```python
from build123d import *

# Parameters (mm, degrees)
SKETCH1_R           = 20
BOSS_EXTRUDE1_DEPTH = 35
CUT_EXTRUDE1_DEPTH  = 15
SKETCH3_R           = 4.1
CUT_EXTRUDE2_DEPTH  = 21
SKETCH4_R           = 2
CUT_EXTRUDE3_DEPTH  = 36
SKETCH5_R           = 17
CUT_EXTRUDE4_DEPTH  = 5
CUT_EXTRUDE5_DEPTH  = 2


with BuildPart() as part:
    # Sketch1 → Boss-Extrude1 (new body)
    with BuildSketch(Plane(origin=(0, 0, 0), x_dir=(1, 0, 0), z_dir=(0, 1, 0))):
        Circle(SKETCH1_R)
    extrude(amount=BOSS_EXTRUDE1_DEPTH)

    # Sketch2 → Cut-Extrude1 (cut)
    with BuildSketch(Plane(origin=(0, 35, 0), x_dir=(1, 0, 0), z_dir=(0, 1, 0))):
        Polygon((-8, 7.5), (-14.495190528, 3.75), (-14.495190528, -3.75), (-8, -7.5), (-1.504809472, -3.75), (-1.504809472, 3.75), align=None)
        Polygon((8, 7.5), (1.504809472, 3.75), (1.504809472, -3.75), (8, -7.5), (14.495190528, -3.75), (14.495190528, 3.75), align=None)
    extrude(amount=-CUT_EXTRUDE1_DEPTH, mode=Mode.SUBTRACT)

    # Sketch3 → Cut-Extrude2 (cut, through all)
    with BuildSketch(Plane(origin=(0, 20, 0), x_dir=(1, 0, 0), z_dir=(0, 1, 0))):
        with Locations((-8, 0)):
            Circle(SKETCH3_R)
        with Locations((8, 0)):
            Circle(SKETCH3_R)
    extrude(amount=-CUT_EXTRUDE2_DEPTH, mode=Mode.SUBTRACT)

    # Sketch4 → Cut-Extrude3 (cut, through all)
    with BuildSketch(Plane(origin=(0, 35, 0), x_dir=(1, 0, 0), z_dir=(0, 1, 0))):
        with Locations((-10.5, 10.5)):
            Circle(SKETCH4_R)
        with Locations((10.5, 10.5)):
            Circle(SKETCH4_R)
        with Locations((10.5, -10.5)):
            Circle(SKETCH4_R)
        with Locations((-10.5, -10.5)):
            Circle(SKETCH4_R)
    extrude(amount=-CUT_EXTRUDE3_DEPTH, mode=Mode.SUBTRACT)

    # Sketch5 → Cut-Extrude4 (cut)
    with BuildSketch(Plane(origin=(0, 35, 0), x_dir=(1, 0, 0), z_dir=(0, 1, 0))):
        Circle(SKETCH5_R)
    extrude(amount=-CUT_EXTRUDE4_DEPTH, mode=Mode.SUBTRACT)

    # Sketch6 → Cut-Extrude5 (cut)
    with BuildSketch(Plane.XZ):
        with BuildLine():
            Line((8, -8.1), (-8, -8.1))
            ThreePointArc((-8, -8.1), (-16.1, 0), (-8, 8.1))
            Line((-8, 8.1), (8, 8.1))
            ThreePointArc((8, 8.1), (16.1, 0), (8, -8.1))
        make_face()
    extrude(amount=-CUT_EXTRUDE5_DEPTH, mode=Mode.SUBTRACT)


solid = part.part
```
CAD build for the part. Positions are in the model's coordinates, mm. A direction names the side the tool comes from. Round coordinates to 2 decimals unless told otherwise and drop trailing zeros. Loops run counter-clockwise (first coordinate to the right, second up) from the corner with the lowest first, then second, coordinate; pieces in that order, holes last. Notation, with made-up numbers: (61.5, 38) - (116.5, 38) arc R15 ccw to (116.5, 49) - close; hole circle Ø9 at (67.5, 52.25). An arc over 180 degrees is marked (long way). Return JSON: item names as keys, results as strings. Group by question number.
Q1. Band-saw the part on C-C on x = -10.5. Give the cut face in (y, z).
Q2. Two-plate mould, pull along Z, no slides. Class faces 1 (the face through (0, 0, 9)), 2 (the face through (9.026, 15.21, 9.148)): +Z half, -Z half, draft (parallel to the pull), parting line (faces both ways), or undercut.
Q3. Drill centre lines: line 1 along X through (y, z) = (10, -10); line 2 along X through (y, z) = (23, -12); line 3 along Z through (x, y) = (12, 28.5). Where is each one in solid material? Low to high. Write a range as [from, to].
Q4. Band-saw the part on D-D on x = 0. Give the cut face in (y, z).
Q5. Band-saw the part on A-A on z = 0. Give the cut face in (x, y), plus the area to 3 significant figures.
Q6. Flat gauge pins, fed straight in: pin 1 Ø9.5 at (x, z) = (-8, 0) entering from +Y; pin 2 Ø3 at (x, z) = (-1, -11.5) entering from +Y; pin 3 Ø10 at (y, z) = (19.5, 8) entering from -X. Where does each tip first touch, or does it go through?
Q7. Tool access for faces 3 (the face through (4.798, 25.07, -5.651)), 4 (the face through (-16.1, 0.99, -0.18)), 5 (the face through (-10.76, 15.21, -12.483)): list every direction of +Z, -Z, +X, -X, +Y, -Y with a clear straight run to the whole face (end or side of a thin tool).
Q8. Band-saw the part on B-B on y = 7. Give the cut face in (x, z).
Solutions:
{
 "1": {"outline": "(0, -17.02) - (35, -17.02) - (35, -13.37) - (30, -13.37) - (30, -12.5) - (0, -12.5) - close; (0, -8.5) - (30, -8.5) - (30, -6.06) - (20, -6.06) - (20, -3.25) - (2, -3.25) - (2, -7.7) - (0, -7.7) - close; (0, 7.7) - (2, 7.7) - (2, 3.25) - (20, 3.25) - (20, 6.06) - (30, 6.06) - (30, 8.5) - (0, 8.5) - close; (0, 12.5) - (30, 12.5) - (30, 13.37) - (35, 13.37) - (35, 17.02) - (0, 17.02) - close"},
 "2": {"face 1": "draft", "face 2": "undercut"},
 "3": {"line 1": "x = [-17.32, -12.44], [-8.56, 8.56], [12.44, 17.32]", "line 2": "x = [-16, -11.82], [-9.18, 9.18], [11.82, 16]", "line 3": "z = [-16, -11.82], [-9.18, -5.19], [5.19, 9.18], [11.82, 16]"},
 "4": {"outline": "(0, -20) - (35, -20) - (35, -17) - (30, -17) - (30, 17) - (35, 17) - (35, 20) - (0, 20) - (0, 8.1) - (2, 8.1) - (2, -8.1) - (0, -8.1) - close"},
 "5": {"outline": "(-20, 0) - (-16.1, 0) - (-16.1, 2) - (-12.1, 2) - (-12.1, 20) - (-14.5, 20) - (-14.5, 30) - (-17, 30) - (-17, 35) - (-20, 35) - close; (-3.9, 2) - (3.9, 2) - (3.9, 20) - (1.5, 20) - (1.5, 30) - (-1.5, 30) - (-1.5, 20) - (-3.9, 20) - close; (12.1, 2) - (16.1, 2) - (16.1, 0) - (20, 0) - (20, 35) - (17, 35) - (17, 30) - (14.5, 30) - (14.5, 20) - (12.1, 20) - close", "area": "611 mm^2"},
 "6": {"pin 1": "stops at y = 20", "pin 2": "stops at y = 30", "pin 3": "stops at x = -19.77"},
 "7": {"face 3": "+Y", "face 4": "-Y", "face 5": "+Y, -Y"},
 "8": {"outline": "circle Ø40 at (0, 0); hole circle Ø4 at (-10.5, -10.5); hole circle Ø4 at (-10.5, 10.5); hole circle Ø8.2 at (-8, 0); hole circle Ø8.2 at (8, 0); hole circle Ø4 at (10.5, -10.5); hole circle Ø4 at (10.5, 10.5)"}
}
